```python
from build123d import *

# Parameters (mm, degrees)
SKETCH1_W                       = 80
SKETCH1_H                       = 40
BOSS_EXTRUDE1_DEPTH             = 6.35
M3X0_5_TAPPED_HOLE2_D           = 2.5
CBORE_FOR_M5_SBHCS1_D           = 5.5
CBORE_FOR_M5_SBHCS1_CBORE_D     = 10.5
CBORE_FOR_M5_SBHCS1_CBORE_DEPTH = 2.75


with BuildPart() as part:
    # Sketch1 → Boss-Extrude1 (new body)
    with BuildSketch(Plane(origin=(0, 0, 0), x_dir=(1, 0, 0), z_dir=(0, 1, 0))):
        Rectangle(SKETCH1_W, SKETCH1_H)
    extrude(amount=BOSS_EXTRUDE1_DEPTH)

    # M3x0.5 Tapped Hole2 (through all)
    with Locations(Plane(origin=(0, 6.35, 0), x_dir=(1, 0, 0), z_dir=(0, 1, 0))):
        with Locations((0, 0), (16, 16), (-16, -16), (-16, 16), (16, -16)):
            Hole(M3X0_5_TAPPED_HOLE2_D / 2)

    # CBORE for M5 SBHCS1 (through all)
    with Locations(Plane(origin=(0, 6.35, 0), x_dir=(1, 0, 0), z_dir=(0, 1, 0))):
        with Locations((10, 10), (30, 12.5), (-30, 12.5), (-10, 10), (30, -12.5), (10, -10), (-10, -10), (-30, -12.5)):
            CounterBoreHole(CBORE_FOR_M5_SBHCS1_D / 2, CBORE_FOR_M5_SBHCS1_CBORE_D / 2, CBORE_FOR_M5_SBHCS1_CBORE_DEPTH)


solid = part.part
```
The listing builds one solid part. Answer for the finished solid, in the listing's coordinates (mm). A direction names the side the tool comes from. Give positions to 0.01 mm unless a question says otherwise; leave off trailing zeros. Loops run counter-clockwise (first coordinate to the right, second up) from the corner with the lowest first, then second, coordinate; pieces in that order, holes last. Notation, with made-up numbers: M 16.5,16.25 L 51.5,16.25 A19 cw 51.5,39.25 Z; hole C -8,25 d5. An arc over 180 degrees is marked long. One line per item, written item: value.
1. Find the intervals of material crossed by probe 1 along Z at (x, y) = (-10, 2.6); probe 2 along X at (y, z) = (2.75, 16); probe 3 along Z at (x, y) = (-10, 5.4), in increasing order.
Found:
probe 1: -20 to -12.75, -7.25 to 7.25, 12.75 to 20
probe 2: -40 to -17.25, -14.75 to 14.75, 17.25 to 40
probe 3: -20 to -15.25, -4.75 to 4.75, 15.25 to 20
2. Section C-C on x = 29.5 is taken. Determine the outline of the cut face in (y, z), plus the area to 3 significant figures.
Found:
outline: M 0,-20 L 6.35,-20 L 6.35,-17.73 L 3.6,-17.73 L 3.6,-15.2 L 0,-15.2 Z; M 0,-9.8 L 3.6,-9.8 L 3.6,-7.27 L 6.35,-7.27 L 6.35,7.27 L 3.6,7.27 L 3.6,9.8 L 0,9.8 Z; M 0,15.2 L 3.6,15.2 L 3.6,17.73 L 6.35,17.73 L 6.35,20 L 0,20 Z
area: 158 mm^2
3. Section A-A on x = 0 is taken. Determine the outline of the cut face in (y, z).
Found:
outline: M 0,-20 L 6.35,-20 L 6.35,-1.25 L 0,-1.25 Z; M 0,1.25 L 6.35,1.25 L 6.35,20 L 0,20 Z
4. This flat-tipped pin is pushed along its axis until it touches: P1, Ø6.5, axis at x = -30, z = -12.5, coming from the +Y side. Where does it stop, or does it pass through?
Found:
P1: y = 3.6
5. Section D-D on z = 16 is taken. Determine the outline of the cut face in (x, y), plus the area to 3 significant figures.
Found:
outline: M -40,0 L -17.25,0 L -17.25,6.35 L -26.09,6.35 L -26.09,3.6 L -33.91,3.6 L -33.91,6.35 L -40,6.35 Z; M -14.75,0 L 14.75,0 L 14.75,6.35 L -14.75,6.35 Z; M 17.25,0 L 40,0 L 40,6.35 L 33.91,6.35 L 33.91,3.6 L 26.09,3.6 L 26.09,6.35 L 17.25,6.35 Z
area: 433 mm^2
6. Section B-B on y = 5.5 is taken. State how many separate pieces and enclosed holes the cut face has, plus the area to 3 significant figures.
Found:
separate pieces: 1
enclosed holes: 13
area: 2,480 mm^2
7. For a pull along X with two mould halves and no side action, classify faces 1 (the face through (-1, 0, 4)), 2 (the face through (40, 3, 0)), 3 (the face through (-16.672, 3.131, -17.054)) as pulls with the +X half, pulls with the -X half, needs draft (parallel to the pull), parting line crosses it, or undercut.
Found:
face 1: needs draft
face 2: pulls with the +X half
face 3: undercut
8. For faces 4 (the face through (12.82, 4.99, -14.43)), 5 (the face through (-1, 3, -20)), determine the directions among +Z, -Z, +X, -X, +Y, -Y from which every point of the face is accessible in a straight line to the end or side of a thin tool.
Found:
face 4: +Y
face 5: -Z, +X, -X, +Y, -Y
